Drawing for the job (mm, zero at the part's lowest x, y, z). Coordinates: 2 decimals unless noted, no trailing zeros. Write each loop counter-clockwise with the first axis right and the second up, starting at its lowest first coordinate (ties: lowest second). Pieces come first, ordered by that corner, then holes. Notation, with made-up numbers: (16, -13.75) -> (58, -13.75) arc R24 ccw to (58, 7.25) -> close; hole circle Ø11 at (10.5, -14.5). An arc over 180 degrees is marked (long way). Write item = value, one per line. Start each with the question number.
Q1. Probe line 1 (Z direction, x = 3.65, y = 8); line 2 (Y direction, x = 2.85, z = 164). List the from-to ranges inside material, lowest first.
Q2. Band-saw the part on A-A, the plane y = 6.5. List the corners of the cut face in (x, z), plus the area to 3 significant figures.
Q3. Band-saw the part on C-C, the plane z = 56. List the corners of the cut face in (x, y), plus the area to 3 significant figures.
Q4. Band-saw the part on B-B, the plane x = 3.6. List the corners of the cut face in (y, z), plus the area to 3 significant figures.
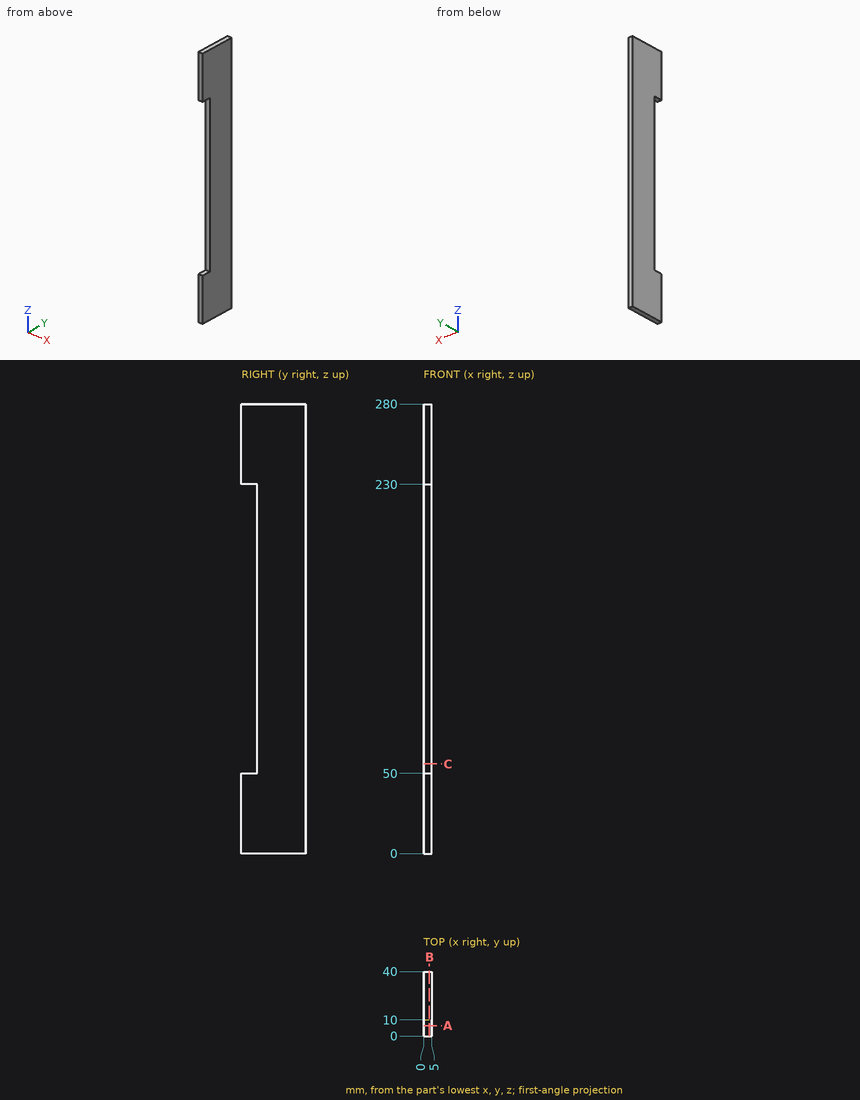
Ans:
q1.line_1 = 0 to 50, 230 to 280
q1.line_2 = 10 to 40
q2.outline = (0, 0) -> (5, 0) -> (5, 50) -> (0, 50) -> close; (0, 230) -> (5, 230) -> (5, 280) -> (0, 280) -> close
q2.area = 500 mm2
q3.outline = (0, 10) -> (5, 10) -> (5, 40) -> (0, 40) -> close
q3.area = 150 mm2
q4.outline = (0, 0) -> (40, 0) -> (40, 280) -> (0, 280) -> (0, 230) -> (10, 230) -> (10, 50) -> (0, 50) -> close
q4.area = 9,400 mm2
